The figure shows three views and two pictorial views of one solid part (mm, origin at its lowest corner). Answer the questions. A direction names the side the tool comes from. Coordinates: 2 decimals unless noted, no trailing zeros. Order: outer loops, then holes, each group sorted by start corner. A loop starts at its lowest first (then second) coordinate and runs counter-clockwise, first axis right, second up. Notation, with made-up numbers: M -23,0 L -13,0 A20 ccw -13,16 Z; hole C -14,-25 d3. An arc over 180 degrees is marked long. Use a Markdown table: item, result.
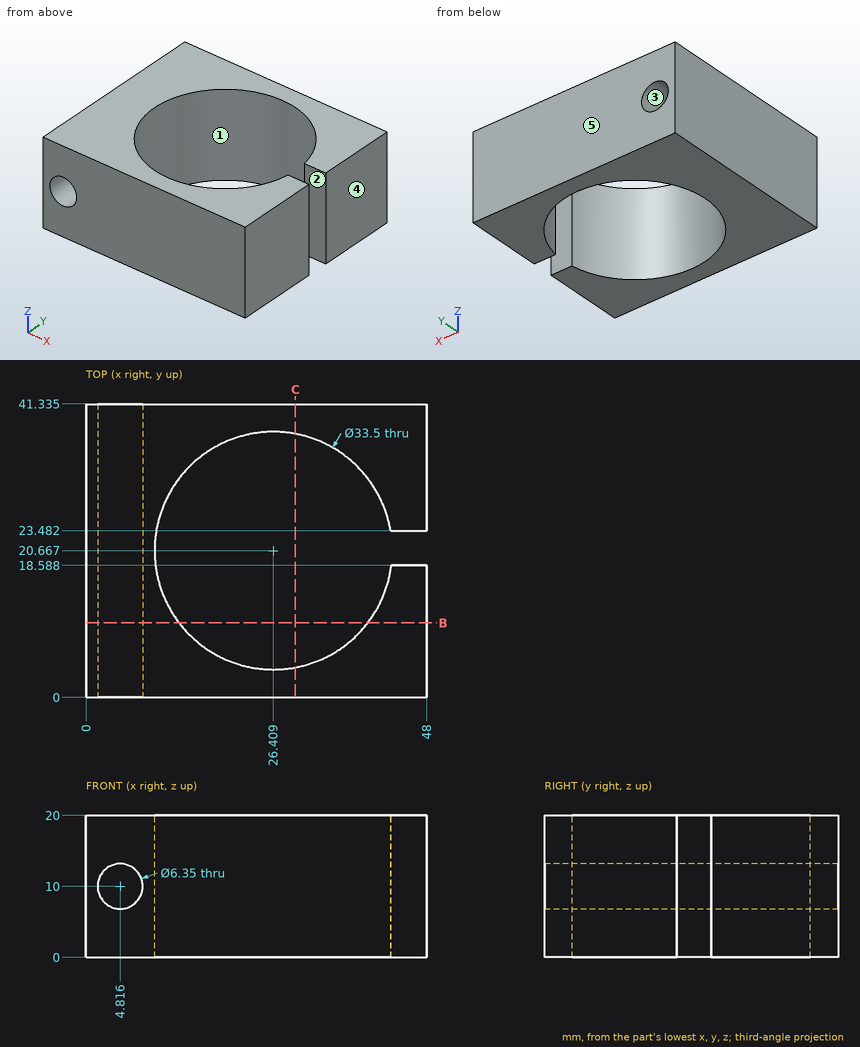
1. A flat-ended cylindrical pin translates along its axis: P1, Ø4, axis at x = 4.82, z = 10, coming from the -Y side. Find the tip coordinate at first contact, or state that the pin passes through.
Answers below:
| item | result |
|---|---|
| P1 | through |
2. Section C-C on x = 29.5 is taken. Determine the outline of the cut face in (y, z) (1 decimal).
Answers below:
| item | result |
|---|---|
| outline | M 0,0 L 4.2,0 L 4.2,20 L 0,20 Z; M 37.1,0 L 41.3,0 L 41.3,20 L 37.1,20 Z |
3. Find the intervals of material crossed by probe 1 along X at (y, z) = (16, 10) (1 decimal); probe 2 along Z at (x, y) = (5, 38.5); probe 3 along X at (y, z) = (26.5, 8.75) (1 decimal), in increasing order.
Answers below:
| item | result |
|---|---|
| probe 1 | 0 to 1.6, 8 to 10.3, 42.5 to 48 |
| probe 2 | 0 to 6.83, 13.17 to 20 |
| probe 3 | 0 to 1.9, 7.7 to 10.7, 42.1 to 48 |
4. For the marked faces 1 and 2, determine the directions among +Z, -Z, +X, -X, +Y, -Y from which every point of the face is accessible in a straight line to the end or side of a thin tool.
Answers below:
| item | result |
|---|---|
| face 1 | +Z, -Z |
| face 2 | +Z, -Z, +X |
5. For a pull along X with two mould halves and no side action, classify the marked faces 3, 4 and 5 as +X half, -X half, draft (parallel to the pull), parting line (faces both ways), or undercut.
Answers below:
| item | result |
|---|---|
| face 3 | undercut |
| face 4 | +X half |
| face 5 | draft |
6. Section B-B on y = 10.5 is taken. Give the number of separate pieces and of enclosed holes in the cut face, then the cut area to 3 significant figures.
Answers below:
| item | result |
|---|---|
| separate pieces | 2 |
| enclosed holes | 1 |
| area | 396 mm² |
